from build123d import *

# Parameters (mm, degrees)
BOSS_EXTRUDE1_START       = -61.874871948
BOSS_EXTRUDE1_DEPTH       = 61.874871948
BOSS_EXTRUDE1_START_2     = 33.418244096
BOSS_EXTRUDE1_2_OUTLINE_W = 41
BOSS_EXTRUDE1_2_OUTLINE_H = 70
BOSS_EXTRUDE1_2_DEPTH     = 4.581755904
SKETCH2_W                 = 31.75
SKETCH2_H                 = 50.8
BOSS_EXTRUDE2_DEPTH       = 12.7
CHAMFER1_SIZE             = 6.35


with BuildPart() as part:
    # Boss-Extrude1: read off the stored shape, not the designer's step
    # Boss-Extrude1 outline → Boss-Extrude1 (new body)
    with BuildSketch(Plane.XY.offset(BOSS_EXTRUDE1_START)):
        with BuildLine():
            Line((-285.755139406, 85.725), (-285.755139406, 92.075))
            Line((-285.755139406, 92.075), (-298.401672666, 92.075))
            ThreePointArc((-298.401672666, 92.075), (-316.362184908, 84.635512242), (-323.801672666, 66.675))
            Line((-323.801672666, 66.675), (-323.801672666, 25.4))
            Line((-323.801672666, 25.4), (-311.15, 25.4))
            Line((-311.15, 25.4), (-311.15, 53.975))
            Line((-311.15, 53.975), (-298.45, 53.975))
            Line((-298.45, 53.975), (-298.45, 85.725))
            Line((-298.45, 85.725), (-285.755139406, 85.725))
        make_face()
    boss_extrude1 = extrude(amount=BOSS_EXTRUDE1_DEPTH)

    # Boss-Extrude1 2 outline → Boss-Extrude1 2 (cut)
    with BuildSketch(Plane(origin=(0, 0, 0), x_dir=(0.9961946980917459, 0, 0.08715574274765299), z_dir=(0.087155742747653, 0, -0.996194698091746)).offset(BOSS_EXTRUDE1_START_2)):
        with Locations((-308.5, -59)):
            Rectangle(BOSS_EXTRUDE1_2_OUTLINE_W, BOSS_EXTRUDE1_2_OUTLINE_H)
    boss_extrude1_2 = extrude(amount=BOSS_EXTRUDE1_2_DEPTH, mode=Mode.SUBTRACT)

    # Mirror1: Boss-Extrude1, Boss-Extrude1 2 across plane
    add(boss_extrude1.mirror(Plane.XY))
    add(boss_extrude1_2.mirror(Plane.XY), mode=Mode.SUBTRACT)

    # Sketch2 → Boss-Extrude2 (add)
    with BuildSketch(Plane(origin=(-298.45, 0, 0), x_dir=(0, 0, -1), z_dir=(1, 0, 0))):
        with Locations((0, 60.325)):
            Rectangle(SKETCH2_W, SKETCH2_H)
    extrude(amount=BOSS_EXTRUDE2_DEPTH)

    # Chamfer1
    chamfer1_edges = [part.edges().sort_by_distance(p)[0] for p in [
        (-292.1, 34.925, -15.875),
        (-292.1, 34.925, 15.875),
        (-292.102569703, 85.725, -15.875),
        (-298.45, 85.725, -37.765943994),
        (-298.45, 69.85, -15.875),
        (-298.45, 85.725, 37.765943994),
        (-292.102569703, 85.725, 15.875),
        (-298.45, 69.85, 15.875),
    ]]
    chamfer(chamfer1_edges, length=CHAMFER1_SIZE)


solid = part.part
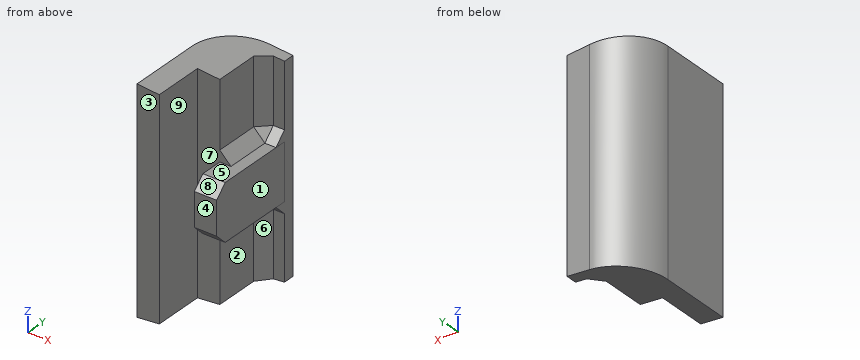
For this review, take the finished solid that the model builds, in its own axes (mm). Face numbers are marked on the shaded views. A direction names the side the tool comes from. Round coordinates to 2 decimals unless told otherwise and drop trailing zeros. Write each loop counter-clockwise with the first axis right and the second up, starting at its lowest first coordinate (ties: lowest second). Pieces come first, ordered by that corner, then holes. Notation, with made-up numbers: (73.5, 16.5) -> (87.5, 16.5) arc R6 ccw to (87.5, 21.5) -> close; hole circle Ø11 at (-25.5, 24). An arc over 180 degrees is marked (long way). Put each result on its own line as item: value.
Q1. Consider section D-D on x = -288.5. State the section outline as (y, z) points (3 decimals), and give its area (3 significant figures).
Determined:
outline: (34.925, -9.525) -> (41.275, -15.875) -> (79.375, -15.875) -> (85.725, -22.225) -> (85.725, -58.786) -> (92.075, -58.786) -> (92.075, 58.786) -> (85.725, 58.786) -> (85.725, 22.225) -> (79.375, 15.875) -> (41.275, 15.875) -> (34.925, 9.525) -> close
area: 2,360 mm^2
Q2. Consider section C-C on y = 63. State the section outline as (x, z) points (3 decimals).
Determined:
outline: (-323.802, -61.875) -> (-298.45, -59.657) -> (-298.45, -22.225) -> (-292.1, -15.875) -> (-285.75, -15.875) -> (-285.75, 15.875) -> (-292.1, 15.875) -> (-298.45, 22.225) -> (-298.45, 59.657) -> (-323.802, 61.875) -> close
Q3. To check wall thickness, follow L1, parallel to Y at x = -287.5, z = -4 (3 decimals); L2, parallel to Y at x = -299, z = -35 (3 decimals); L3, parallel to X at y = 66.5, z = 41. State the ranges of each line that lie inside material, in increasing order. Write a range as [from, to].
Determined:
L1: y = [34.925, 92.075]
L2: y = [53.975, 92.068]
L3: x = [-323.8, -298.45]
Q4. Consider section B-B on z = 30.5. State the section outline as (x, y) points (3 decimals).
Determined:
outline: (-323.802, 25.4) -> (-311.15, 25.4) -> (-311.15, 53.975) -> (-298.45, 53.975) -> (-298.45, 79.375) -> (-292.1, 85.725) -> (-285.755, 85.725) -> (-285.755, 92.075) -> (-298.402, 92.075) arc R25.4 ccw to (-323.802, 66.675) -> close
Q5. Consider section A-A on y = 43. State the section outline as (x, z) points (3 decimals).
Determined:
outline: (-323.802, -61.875) -> (-311.15, -60.768) -> (-311.15, 60.768) -> (-323.802, 61.875) -> close; (-298.45, -15.875) -> (-285.75, -15.875) -> (-285.75, 15.875) -> (-298.45, 15.875) -> close
Q6. The part is to be moulded in two halves that separate along X. For the marked faces 6, 7, 8 and 9, say which applies: released by +X, released by -X, zero draft, split by the parting line, or undercut.
Determined:
face 6: released by +X
face 7: undercut
face 8: zero draft
face 9: undercut
Q7. Machinability: for the marked faces 1, 2, 3, 4 and 5, which of the approach directions +Z, -Z, +X, -X, +Y, -Y give a long, thin tool a straight path to every point of the face, cutting with its end or side? Answer none if there is none.
Determined:
face 1: +Z, -Z, +X, +Y, -Y
face 2: -Z, +X, -Y
face 3: +Z, -Z, +X, -X, -Y
face 4: +Z, -Z, +X, -Y
face 5: +Z, +X, -Y
Q8. Clearance check with flat-ended pins moving along their axes: pin 1 Ø1.9 at (x, z) = (-288.5, 36) entering from -Y (3 decimals); pin 2 Ø4 at (x, y) = (-303, 74.5) entering from +Z; pin 3 Ø3 at (x, z) = (-300.5, 23) entering from +Y. State where each tip first meets the part, or that it passes through.
Determined:
pin 1: stops at y = 85.725
pin 2: stops at z = 60.23
pin 3: stops at y = 92.07
